Verification items for the finished model (mm, model axes). A direction names the side the tool comes from. Round coordinates to 2 decimals unless told otherwise and drop trailing zeros. Order: outer loops, then holes, each group sorted by start corner. A loop starts at its lowest first (then second) coordinate and runs counter-clockwise, first axis right, second up. Notation, with made-up numbers: (13, 17) -> (44, 17) arc R30 cw to (44, 46) -> close; hole circle Ø6 at (-31, 37.25). An arc over 180 degrees is marked (long way). Put each result on its own line as item: value.
from build123d import *

# Parameters (mm, degrees)
F1_DEPTH = 10


with BuildPart() as f1:
    # F0 (on Top) → F1 (new body)
    with BuildSketch(Plane.XY):
        with BuildLine():
            ThreePointArc((0, -2), (-1.26591, 1.548377), (1.960106, -0.397472))
            ThreePointArc((1.960106, -0.397472), (2.007714, -0.729789), (2.254767, -0.957092))
            Line((2.254767, -0.957092), (3.188722, -1.353532))
            ThreePointArc((3.188722, -1.353532), (3.604109, -1.342268), (3.867529, -1.020891))
            ThreePointArc((3.867529, -1.020891), (-2.440946, 3.168877), (0, -4))
            ThreePointArc((0, -4), (1.26591, -7.548377), (-1.960106, -5.602528))
            ThreePointArc((-1.960106, -5.602528), (-2.007714, -5.270211), (-2.254767, -5.042908))
            Line((-2.254767, -5.042908), (-3.188722, -4.646468))
            ThreePointArc((-3.188722, -4.646468), (-3.604109, -4.657732), (-3.867529, -4.979109))
            ThreePointArc((-3.867529, -4.979109), (2.440946, -9.168877), (0, -2))
        make_face()
    extrude(amount=F1_DEPTH)


solid = f1.part
Item 1: Section check C-C on x = 2.75. Record the boundary of the cut face in (y, z).
Check sheet entries:
outline: (-8.9, 0) -> (-3.1, 0) -> (-3.1, 10) -> (-8.9, 10) -> close; (-1.17, 0) -> (2.9, 0) -> (2.9, 10) -> (-1.17, 10) -> close
Item 2: Section check A-A on x = 0. Record the boundary of the cut face in (y, z).
Check sheet entries:
outline: (-10, 0) -> (-8, 0) -> (-8, 10) -> (-10, 10) -> close; (-4, 0) -> (-2, 0) -> (-2, 10) -> (-4, 10) -> close; (2, 0) -> (4, 0) -> (4, 10) -> (2, 10) -> close
Item 3: Material ranges on L1, parallel to Y at x = -0.75, z = 9.25; L2, parallel to Y at x = 1.75, z = 8; L3, parallel to X at y = 0, z = 2.75, recorded low to high. Write a range as [from, to].
Check sheet entries:
L1: y = [-9.93, -7.85], [-3.93, -1.85], [1.85, 3.93]
L2: y = [-9.6, -6.97], [-5.03, -2.4], [0.97, 3.6]
L3: x = [-4, -2], [2, 4]
Item 4: Section check B-B on y = 0. Record the boundary of the cut face in (x, z).
Check sheet entries:
outline: (-4, 0) -> (-2, 0) -> (-2, 10) -> (-4, 10) -> close; (2, 0) -> (4, 0) -> (4, 10) -> (2, 10) -> close
Item 5: Section check D-D on z = 6.5. Record the boundary of the cut face in (x, y), then the cut area to 3 significant figures.
Check sheet entries:
outline: (-3.87, -4.98) arc R4 ccw (long way) to (0, -2) arc R2 cw (long way) to (1.96, -0.4) arc R0.5 ccw to (2.25, -0.96) -> (3.19, -1.35) arc R0.5 ccw to (3.87, -1.02) arc R4 ccw (long way) to (0, -4) arc R2 cw (long way) to (-1.96, -5.6) arc R0.5 ccw to (-2.25, -5.04) -> (-3.19, -4.65) arc R0.5 ccw to start
area: 61.2 mm^2
Item 6: Gauge pin test, flat ends, axial feed: pin 1 Ø1 at (y, z) = (-2.5, 8.5) entering from -X; pin 2 Ø1.5 at (y, z) = (1.5, 8.5) entering from -X. Record the tip position at first contact, or that the pin passes through.
Check sheet entries:
pin 1: stops at x = -3.46
pin 2: stops at x = -3.93
Item 7: Release check for a two-part mould opening along X. For faces 3 (the cylindrical face through (2.33, -9.25, 4.93)), 4 (the flat face through (2.715, -1.153, 4.93)), 5 (the flat face through (0, -3, 0)) record: +X half, -X half, draft (parallel to the pull), parting line (faces both ways), or undercut.
Check sheet entries:
face 3: parting line
face 4: undercut
face 5: draft
Item 8: Tool access check on faces 1 (the flat face through (0, -3, 10)), 2 (the flat face through (-2.715, -4.847, 4.93)). Record the directions out of +Z, -Z, +X, -X, +Y, -Y that give a thin tool (end or side, any length) a straight path to the whole face; none if there is none.
Check sheet entries:
face 1: +Z, +X, -X, +Y, -Y
face 2: +Z, -Z
